Geometry check sheet. Reference: the model listing, model coordinates, mm. Face numbers are marked on the shaded views. A direction names the side the tool comes from. Give positions to 0.01 mm unless a question says otherwise; leave off trailing zeros. Write each loop counter-clockwise with the first axis right and the second up, starting at its lowest first coordinate (ties: lowest second). Pieces come first, ordered by that corner, then holes.
(1) Tool access check on the marked faces 3 and 4. Record the directions out of +Z, -Z, +X, -X, +Y, -Y that give a thin tool (end or side, any length) a straight path to the whole face; none if there is none.
(2) Cross-section at B-B (x = 299). Record the boundary of the cut face in (y, z), and give its area (3 significant figures).
(3) Cross-section at C-C (z = 114.5). Record the boundary of the cut face in (x, y).
(4) Thickness scan on line 1 along Z through (x, y) = (225, 11.5); line 2 along Z through (x, y) = (159.81, 6); line 3 along Z through (x, y) = (-78, 19). Record the ranges inside material, lowest first.
(5) Cross-section at A-A (y = 5.5). Record the boundary of the cut face in (x, z), and give its area (3 significant figures).
(6) Mould release check, pull along X, two halves, no side actions. Record for the marked faces 1 and 2: +X half, -X half, draft (parallel to the pull), parting line (faces both ways), or undercut.
(7) Cross-section at D-D (z = -39). Record the boundary of the cut face in (x, y), and give its area (3 significant figures).
(8) Depth check by flat-ended pin: P1, Ø10, axis at x = -85.5, z = -45.5, coming from the -Y side; P2, Ø1, axis at x = -40, y = 9.5, coming from the +Z side; P3, Ø11, axis at y = 18, z = 52.5, coming from the -X side; P4, Ø4, axis at x = 199.5, z = 123.5, coming from the +Y side. Enter the tip coordinate at first touch or a pass-through.
```python
from build123d import *

# Parameters (mm, degrees)
SKETCH1_R           = 61.5
SKETCH1_W           = 390
SKETCH1_H           = 302.5
BOSS_EXTRUDE1_DEPTH = 25
SKETCH1_4_W         = 390
SKETCH1_4_H         = 302.5
SKETCH1_4_R         = 5
SKETCH1_4_R_2       = 61.5
BOSS_EXTRUDE2_DEPTH = 15
SKETCH3_R           = 3.5
CUT_EXTRUDE1_DEPTH  = 26


with BuildPart() as part:
    # Sketch1 → Boss-Extrude1 (new body)
    with BuildSketch(Plane(origin=(0, 0, 0), x_dir=(1, 0, 0), z_dir=(0, 1, 0))):
        with BuildLine():
            Line((0, 188.75), (450, 188.75))
            Line((450, 188.75), (450, -188.75))
            Line((450, -188.75), (0, -188.75))
            Line((0, -188.75), (0, -70.5))
            Line((0, -70.5), (-78, -70.5))
            ThreePointArc((-78, -70.5), (-148.5, 0), (-78, 70.5))
            Line((-78, 70.5), (0, 70.5))
            Line((0, 70.5), (0, 188.75))
        make_face()
        with Locations((-78, 0)):
            Circle(SKETCH1_R, mode=Mode.SUBTRACT)
        with Locations((240, 0)):
            Rectangle(SKETCH1_W, SKETCH1_H, mode=Mode.SUBTRACT)
    extrude(amount=BOSS_EXTRUDE1_DEPTH)

    # Sketch1<4> → Boss-Extrude2 (add)
    with BuildSketch(Plane(origin=(0, 0, 0), x_dir=(1, 0, 0), z_dir=(0, 1, 0))):
        with Locations((240, 0)):
            Rectangle(SKETCH1_4_W, SKETCH1_4_H)
        with Locations((225, 136.25)):
            Circle(SKETCH1_4_R, mode=Mode.SUBTRACT)
        with Locations((225, -136.25)):
            Circle(SKETCH1_4_R, mode=Mode.SUBTRACT)
        with Locations((-78, 0)):
            Circle(SKETCH1_4_R_2)
    extrude(amount=BOSS_EXTRUDE2_DEPTH)

    # Sketch3 → Cut-Extrude1 (cut, through all)
    with BuildSketch(Plane(origin=(0, 25, 0), x_dir=(1, 0, 0), z_dir=(0, 1, 0))):
        with Locations((159.81, -170)):
            Circle(SKETCH3_R)
        with Locations((204.81, -170)):
            Circle(SKETCH3_R)
        with Locations((204.81, 170)):
            Circle(SKETCH3_R)
        with Locations((159.81, 170)):
            Circle(SKETCH3_R)
    extrude(amount=-CUT_EXTRUDE1_DEPTH, mode=Mode.SUBTRACT)


solid = part.part
```
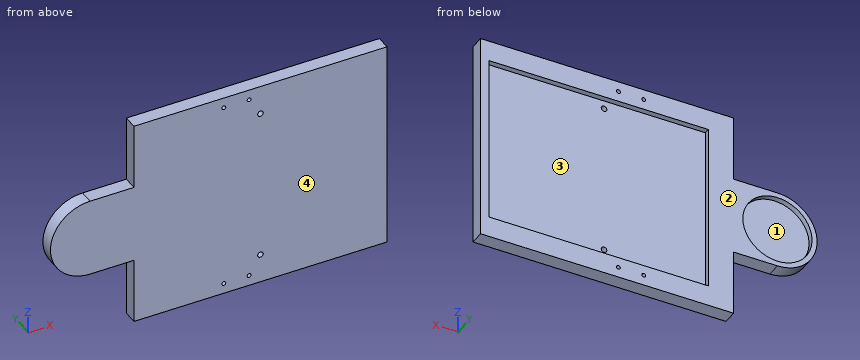
Reply:
1. face 3: +Y
1. face 4: +Z, -Z, +X, -X, -Y
2. outline: (0, -188.75) - (25, -188.75) - (25, -151.25) - (15, -151.25) - (15, 151.25) - (25, 151.25) - (25, 188.75) - (0, 188.75) - close
2. area: 6,410 mm2
3. outline: (0, 0) - (450, 0) - (450, 25) - (435, 25) - (435, 15) - (45, 15) - (45, 25) - (0, 25) - close
4. line 1: z = -188.75 to -141.25, -131.25 to 131.25, 141.25 to 188.75
4. line 2: z = -188.75 to -173.5, -166.5 to 166.5, 173.5 to 188.75
4. line 3: z = -70.5 to -61.5, 61.5 to 70.5
5. outline: (-78, -70.5) - (0, -70.5) - (0, -188.75) - (450, -188.75) - (450, 188.75) - (0, 188.75) - (0, 70.5) - (-78, 70.5) arc R70.5 ccw to start; hole circle Ø7 at (159.81, -170); hole circle Ø7 at (159.81, 170); hole circle Ø7 at (204.81, -170); hole circle Ø7 at (204.81, 170); hole circle Ø10 at (225, -136.25); hole circle Ø10 at (225, 136.25)
5. area: 188,000 mm2
6. face 1: undercut
6. face 2: draft
7. outline: (-136.73, 0) - (450, 0) - (450, 25) - (435, 25) - (435, 15) - (45, 15) - (45, 25) - (-30.45, 25) - (-30.45, 15) - (-125.55, 15) - (-125.55, 25) - (-136.73, 25) - close
7. area: 9,820 mm2
8. P1: stops at y = 0
8. P2: stops at z = 70.5
8. P3: stops at x = -130.55
8. P4: stops at y = 15
